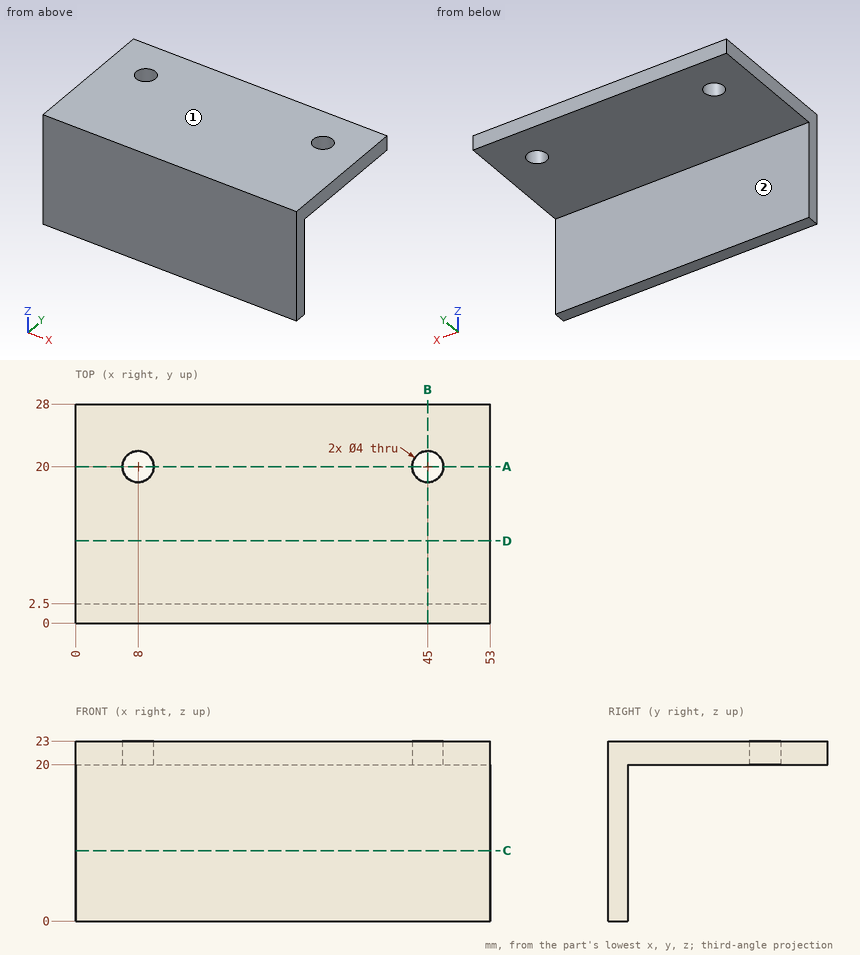
For this review, use the dimensioned drawing (mm, ordinates from the lowest corner) and the shaded views. A direction names the side the tool comes from. Round coordinates to 2 decimals unless told otherwise and drop trailing zeros. Write each loop counter-clockwise with the first axis right and the second up, starting at its lowest first coordinate (ties: lowest second). Pieces come first, ordered by that corner, then holes. Notation, with made-up numbers: M 49.25,-32 L 77.25,-32 A27 ccw 77.25,-10 Z; hole C -17,75 d2. An arc over 180 degrees is marked long. Write item = value, one per line. Start each with the question number.
(1) Clearance check with flat-ended pins moving along their axes: pin 1 Ø1.5 at (x, z) = (44.5, 10) entering from +Y; pin 2 Ø5 at (x, y) = (8, 20) entering from -Z. State where each tip first meets the part, or that it passes through.
(2) We need section A-A (y = 20). Give the boundary of the cut face in (x, z), then the cut area to 3 significant figures.
(3) We need section D-D (y = 10.5). Give the boundary of the cut face in (x, z), then the cut area to 3 significant figures.
(4) For line 1 along X through (y, z) = (20, 21.6); line 2 along Y through (x, z) = (45, 21.5); line 3 along Y through (x, z) = (25.5, 4.75), list the stretches that pass through material, from the lowest coordinate up.
(5) For the marked faces 1 and 2, list the 3-axis set-ups (+Z, -Z, +X, -X, +Y, -Y) from which the entire face can be reached by the end or side of a thin tool; tool diameter is ignored.
(6) We need section C-C (z = 9). Give the boundary of the cut face in (x, y), then the cut area to 4 significant figures.
(7) We need section B-B (x = 45). Give the boundary of the cut face in (y, z), then the cut area to 3 significant figures.
Results found:
q1.pin_1 = 2.5
q1.pin_2 = 20
q2.outline = M 0,20 L 6,20 L 6,23 L 0,23 Z; M 10,20 L 43,20 L 43,23 L 10,23 Z; M 47,20 L 53,20 L 53,23 L 47,23 Z
q2.area = 135 mm²
q3.outline = M 0,20 L 53,20 L 53,23 L 0,23 Z
q3.area = 159 mm²
q4.line_1 = 0 to 6, 10 to 43, 47 to 53
q4.line_2 = 0 to 18, 22 to 28
q4.line_3 = 0 to 2.5
q5.face_1 = +Z, +X, -X, +Y, -Y
q5.face_2 = -Z, +X, -X, +Y
q6.outline = M 0,0 L 53,0 L 53,2.5 L 0,2.5 Z
q6.area = 132.5 mm²
q7.outline = M 0,0 L 2.5,0 L 2.5,20 L 18,20 L 18,23 L 0,23 Z; M 22,20 L 28,20 L 28,23 L 22,23 Z
q7.area = 122 mm²
